Verification items for the finished model (mm, model axes). Coordinates: 2 decimals unless noted, no trailing zeros. Order: outer loops, then holes, each group sorted by start corner. A loop starts at its lowest first (then second) coordinate and runs counter-clockwise, first axis right, second up. Notation, with made-up numbers: M -28.75,38.5 L 5.25,38.5 A30 cw 5.25,76.5 Z; hole C -39.5,62.5 d5. An arc over 180 degrees is marked long. Write item = value, one per line.
```python
from build123d import *

# Parameters (mm, degrees)
F0_W     = 12
F0_H     = 30
F1_DEPTH = 9.5
F3_D     = 6
F4_D     = 6


with BuildPart() as f1:
    # F0 (on Right) → F1 (new body)
    with BuildSketch(Plane.YZ):
        with Locations((-6, 15)):
            Rectangle(F0_W, F0_H)
    extrude(amount=F1_DEPTH)

    # F3 (through all)
    with Locations(Plane.YZ.offset(9.5)):
        with Locations((-6, 9)):
            Hole(F3_D / 2)

    # F4 (through all)
    with Locations(Plane.YZ.offset(9.5)):
        with Locations((-6, 21)):
            Hole(F4_D / 2)


solid = f1.part
```
Item 1: Release check for a two-part mould opening along Z. For faces 1 (the flat face through (5, -6, 0)), 2 (the flat face through (9.5, -6, 15)), 3 (the cylindrical face through (4.68, -8.77, 19.85)) record: pulls with the +Z half, pulls with the -Z half, needs draft (parallel to the pull), parting line crosses it, or undercut.
Report:
face_1 = pulls with the -Z half
face_2 = needs draft
face_3 = undercut
Item 2: Sectioned sample at D-D, the plane z = 11. Enter the section's corners in (x, y), then the cut area to 3 significant figures.
Report:
outline = M 0,-12 L 9.5,-12 L 9.5,-8.24 L 0,-8.24 Z; M 0,-3.76 L 9.5,-3.76 L 9.5,0 L 0,0 Z
area = 71.5 mm^2
Item 3: Sectioned sample at C-C, the plane x = 4.25. Enter the section's corners in (y, z).
Report:
outline = M -12,0 L 0,0 L 0,30 L -12,30 Z; hole C -6,9 d6; hole C -6,21 d6
Item 4: Sectioned sample at B-B, the plane z = 21. Enter the section's corners in (x, y), then the cut area to 3 significant figures.
Report:
outline = M 0,-12 L 9.5,-12 L 9.5,-9 L 0,-9 Z; M 0,-3 L 9.5,-3 L 9.5,0 L 0,0 Z
area = 57.0 mm^2
Item 5: Sectioned sample at A-A, the plane y = -6. Enter the section's corners in (x, z).
Report:
outline = M 0,0 L 9.5,0 L 9.5,6 L 0,6 Z; M 0,12 L 9.5,12 L 9.5,18 L 0,18 Z; M 0,24 L 9.5,24 L 9.5,30 L 0,30 Z
Item 6: Scan lines: L1, parallel to Z at x = 6.5, y = -6; L2, parallel to Z at x = 4.5, y = -7.75; L3, parallel to Y at x = 0.5, z = 19.5. Record each from-to range of solid material in increasing order. Write a range as from..to.
Report:
L1 = 0..6, 12..18, 24..30
L2 = 0..6.56, 11.44..18.56, 23.44..30
L3 = -12..-8.6, -3.4..0
Item 7: Gauge pin test, flat end, axial feed: pin 1 (5 mm diameter, centred on y = -7.5, z = 17, fed in from -X). Record the tip position at first contact, or that the pin passes through.
Report:
pin_1 = 0
